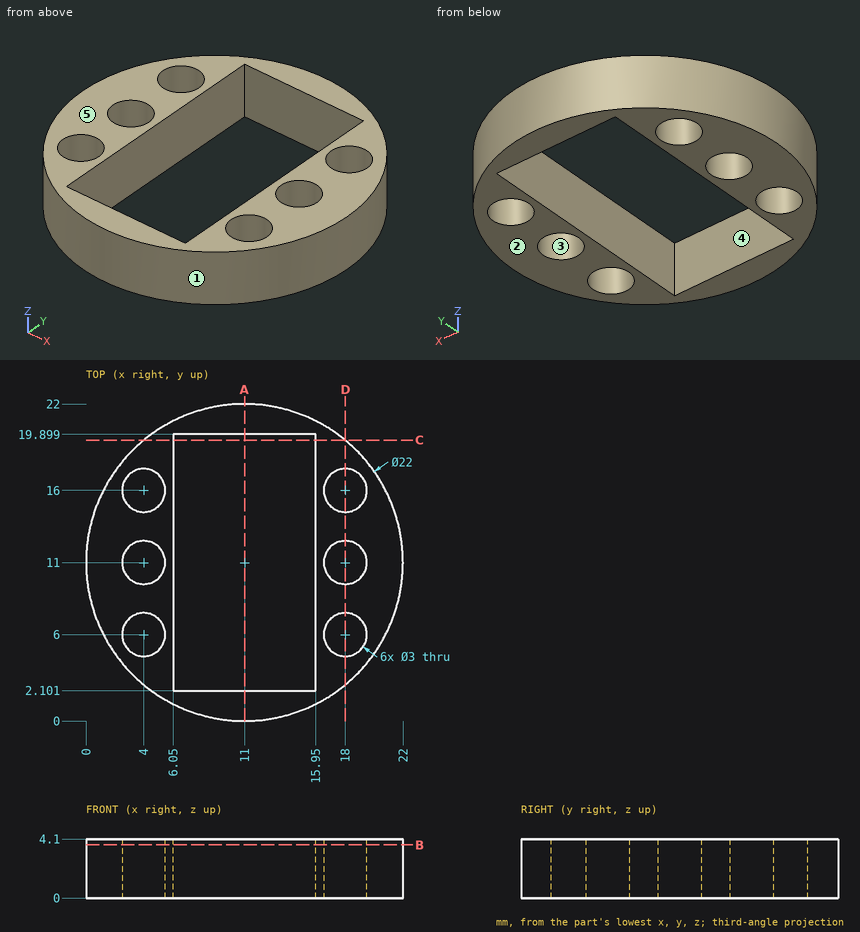
Job drawing, mm, ordinate dimensions from the low corner. One solid piece. A direction names the side the tool comes from. Coordinates: 2 decimals unless noted, no trailing zeros. Write each loop counter-clockwise with the first axis right and the second up, starting at its lowest first coordinate (ties: lowest second). Pieces come first, ordered by that corner, then holes.
Item 1: Which spindle directions (+Z, -Z, +X, -X, +Y, -Y) get a long thin tool onto all of the face, cutting with end or side? Do the marked faces 4 and 5. Say none if no direction does.
Item 2: Slice it at D-D (x = 18). Write the cut outline in (y, z) (1 decimal).
Item 3: Mould opens along Y. For the marked faces 1, 2 and 3 say: released by +Y, released by -Y, zero draft, split by the parting line, or undercut.
Item 4: Pin check, flat tips, straight feed: pin 1 (2 mm diameter, centred on y = 9, z = 3, fed in from +X); pin 2 (1.2 mm diameter, centred on x = 12, z = 1.5, fed in from +Y); pin 3 (1.2 mm diameter, centred on x = 12, z = 1, fed in from -Y). Stop position of each tip, or through.
Item 5: Slice it at A-A (x = 11). Write the cut outline in (y, z).
Item 6: Slice it at B-B (z = 3.7). Write the cut outline in (x, y).
Item 7: Probe line 1 (Y direction, x = 18.25, z = 1.95); line 2 (Y direction, x = 4, z = 1.5) (1 decimal); line 3 (X direction, y = 11.25, z = 3). List the from-to ranges inside material, lowest first.
Item 8: Slice it at C-C (y = 19.5). Write the cut outline in (x, z).
Results found:
1. face 4: +Z, -Z
1. face 5: +Z, +X, -X, +Y, -Y
2. outline: (2.5, 0) - (4.5, 0) - (4.5, 4.1) - (2.5, 4.1) - close; (7.5, 0) - (9.5, 0) - (9.5, 4.1) - (7.5, 4.1) - close; (12.5, 0) - (14.5, 0) - (14.5, 4.1) - (12.5, 4.1) - close; (17.5, 0) - (19.5, 0) - (19.5, 4.1) - (17.5, 4.1) - close
3. face 1: split by the parting line
3. face 2: zero draft
3. face 3: undercut
4. pin 1: stops at x = 21.95
4. pin 2: stops at y = 21.99
4. pin 3: stops at y = 0.01
5. outline: (0, 0) - (2.1, 0) - (2.1, 4.1) - (0, 4.1) - close; (19.9, 0) - (22, 0) - (22, 4.1) - (19.9, 4.1) - close
6. outline: circle Ø22 at (11, 11); hole circle Ø3 at (4, 6); hole circle Ø3 at (4, 11); hole circle Ø3 at (4, 16); hole (6.05, 2.1) - (15.95, 2.1) - (15.95, 19.9) - (6.05, 19.9) - close; hole circle Ø3 at (18, 6); hole circle Ø3 at (18, 11); hole circle Ø3 at (18, 16)
7. line 1: y = 2.73 to 4.52, 7.48 to 9.52, 12.48 to 14.52, 17.48 to 19.27
7. line 2: y = 2.5 to 4.5, 7.5 to 9.5, 12.5 to 14.5, 17.5 to 19.5
7. line 3: x = 0 to 2.52, 5.48 to 6.05, 15.95 to 16.52, 19.48 to 22
8. outline: (4.02, 0) - (6.05, 0) - (6.05, 4.1) - (4.02, 4.1) - close; (15.95, 0) - (17.98, 0) - (17.98, 4.1) - (15.95, 4.1) - close
